CAD build for the part. Positions are in the model's coordinates, mm. Face numbers are marked on the shaded views. A direction names the side the tool comes from. Coordinates: 2 decimals unless noted, no trailing zeros. Loops run counter-clockwise (first coordinate to the right, second up) from the corner with the lowest first, then second, coordinate; pieces in that order, holes last. Notation, with made-up numbers: (8.5, 20) -> (27.5, 20) arc R22 ccw to (27.5, 29) -> close; hole circle Ø8 at (-1, 36.5). An arc over 180 degrees is marked (long way). Write item = value, one per line. Start each with the question number.
(1) Pull direction X, two halves, no side cores. Call the marked faces 6, 7 and 8: +X half, -X half, draft (parallel to the pull), parting line (faces both ways), or undercut.
(2) Drill centre lines: line 1 (Y direction, x = 0, z = 144); line 2 (Z direction, x = -84.5, y = 81); line 3 (Z direction, x = -24.5, y = -29.5). Where is each one in solid material? Low to high. Write a range as from..to.
(3) Flat gauge pins, fed straight in: P1, Ø6, axis at y = 99, z = 131, coming from the -X side; P2, Ø6, axis at y = 99.5, z = 132, coming from the +X side; P3, Ø5, axis at x = -69.5, y = 20.5, coming from the +Z side. Where does each tip first touch, or does it go through?
(4) Band-saw the part on C-C (z = 39.5). Write the cut outline in (x, y).
(5) Band-saw the part on A-A (x = 0). Count the separate pieces of the cut face and the enclosed holes in it, and give its area (3 significant figures).
(6) Tool access for the marked faces 1, 2, 3, 4 and 5: list every direction of +Z, -Z, +X, -X, +Y, -Y with a clear straight run to the whole face (end or side of a thin tool).
```python
from build123d import *

# Parameters (mm, degrees)
F4_DEPTH = 20
F5_R     = 5
F7_D     = 15


with BuildPart() as f1:
    # F0 (on Front) → F1 (revolve)
    with BuildSketch(Plane.XZ):
        Polygon((-37.5, 0), (-37.5, 135), (-75, 135), (-75, 150), (-125, 150), (-125, 110), (-75, 110), (-67.9289321881, 102.9289321881), (-49.7797843479, 0), align=None)
    revolve(axis=Axis((0, 0, 75), (0, 0, 1)))

    # F3 (on offset) → F4 (cut)
    with BuildSketch(Plane.XY.offset(140)):
        with BuildLine():
            ThreePointArc((-61.5454401063, 58.6272871803), (-42.5, 73.6121593217), (-20, 82.6135582093))
            Line((-20, 82.6135582093), (-20, 123.3896267925))
            ThreePointArc((-20, 123.3896267925), (-62.5, 108.2531754731), (-96.8585513658, 79.015321472))
            Line((-96.8585513658, 79.015321472), (-61.5454401063, 58.6272871803))
        make_face()
        with BuildLine():
            ThreePointArc((20, 82.6135582093), (42.5, 73.6121593217), (61.5454401063, 58.6272871803))
            Line((61.5454401063, 58.6272871803), (96.8585513658, 79.015321472))
            ThreePointArc((96.8585513658, 79.015321472), (62.5, 108.2531754731), (20, 123.3896267925))
            Line((20, 123.3896267925), (20, 82.6135582093))
        make_face()
        with BuildLine():
            ThreePointArc((81.5454401063, 23.986271029), (84.1319273791, 12.1168806004), (85, 0))
            ThreePointArc((85, 0), (84.1319273791, -12.1168806004), (81.5454401063, -23.986271029))
            Line((81.5454401063, -23.986271029), (116.8585513658, -44.3743053206))
            ThreePointArc((116.8585513658, -44.3743053206), (122.9477916043, -22.5574940904), (125, 0))
            ThreePointArc((125, 0), (122.9477916043, 22.5574940904), (116.8585513658, 44.3743053206))
            Line((116.8585513658, 44.3743053206), (81.5454401063, 23.986271029))
        make_face()
        with BuildLine():
            Line((96.8585513658, -79.015321472), (61.5454401063, -58.6272871803))
            ThreePointArc((61.5454401063, -58.6272871803), (42.5, -73.6121593217), (20, -82.6135582093))
            Line((20, -82.6135582093), (20, -123.3896267925))
            ThreePointArc((20, -123.3896267925), (62.5, -108.2531754731), (96.8585513658, -79.015321472))
        make_face()
        with BuildLine():
            Line((-20, -123.3896267925), (-20, -82.6135582093))
            ThreePointArc((-20, -82.6135582093), (-42.5, -73.6121593217), (-61.5454401063, -58.6272871803))
            Line((-61.5454401063, -58.6272871803), (-96.8585513658, -79.015321472))
            ThreePointArc((-96.8585513658, -79.015321472), (-62.5, -108.2531754731), (-20, -123.3896267925))
        make_face()
        with BuildLine():
            ThreePointArc((-81.5454401063, -23.986271029), (-85, 0), (-81.5454401063, 23.986271029))
            Line((-81.5454401063, 23.986271029), (-116.8585513658, 44.3743053206))
            ThreePointArc((-116.8585513658, 44.3743053206), (-125, 0), (-116.8585513658, -44.3743053206))
            Line((-116.8585513658, -44.3743053206), (-81.5454401063, -23.986271029))
        make_face()
    extrude(amount=-F4_DEPTH, mode=Mode.SUBTRACT)

    # F5
    f5_edges = [f1.edges().sort_by_distance(p)[0] for p in [
        (125, 0, 150),
        (125, 0, 110),
        (49.779784, 0, 0),
    ]]
    fillet(f5_edges, radius=F5_R)

    # F7 (through all)
    with Locations(Plane.XY.offset(150)):
        with Locations((86.6025403784, 50), (86.6025403784, -50), (0, -100), (-86.6025403784, -50), (-86.6025403784, 50), (0, 100)):
            Hole(F7_D / 2)


solid = f1.part
```
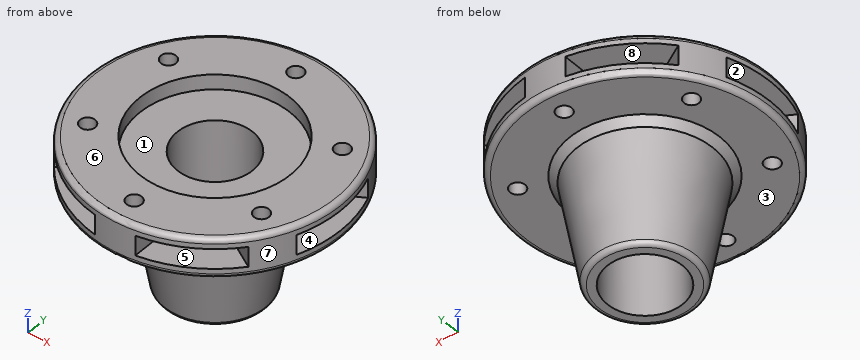
Findings below:
q1.face_6 = draft
q1.face_7 = parting line
q1.face_8 = undercut
q2.line_1 = -125..-107.5, -92.5..-75, 75..92.5, 107.5..125
q2.line_2 = 110..120, 140..150
q2.line_3 = 0..135
q3.P1 = -20
q3.P2 = 20
q3.P3 = 135
q4.outline = circle Ø113.49 at (0, 0); hole circle Ø75 at (0, 0)
q5.separate_pieces = 4
q5.enclosed_holes = 0
q5.area = 9,520 mm²
q6.face_1 = +Z
q6.face_2 = -X
q6.face_3 = -Z
q6.face_4 = +X
q6.face_5 = -Y
